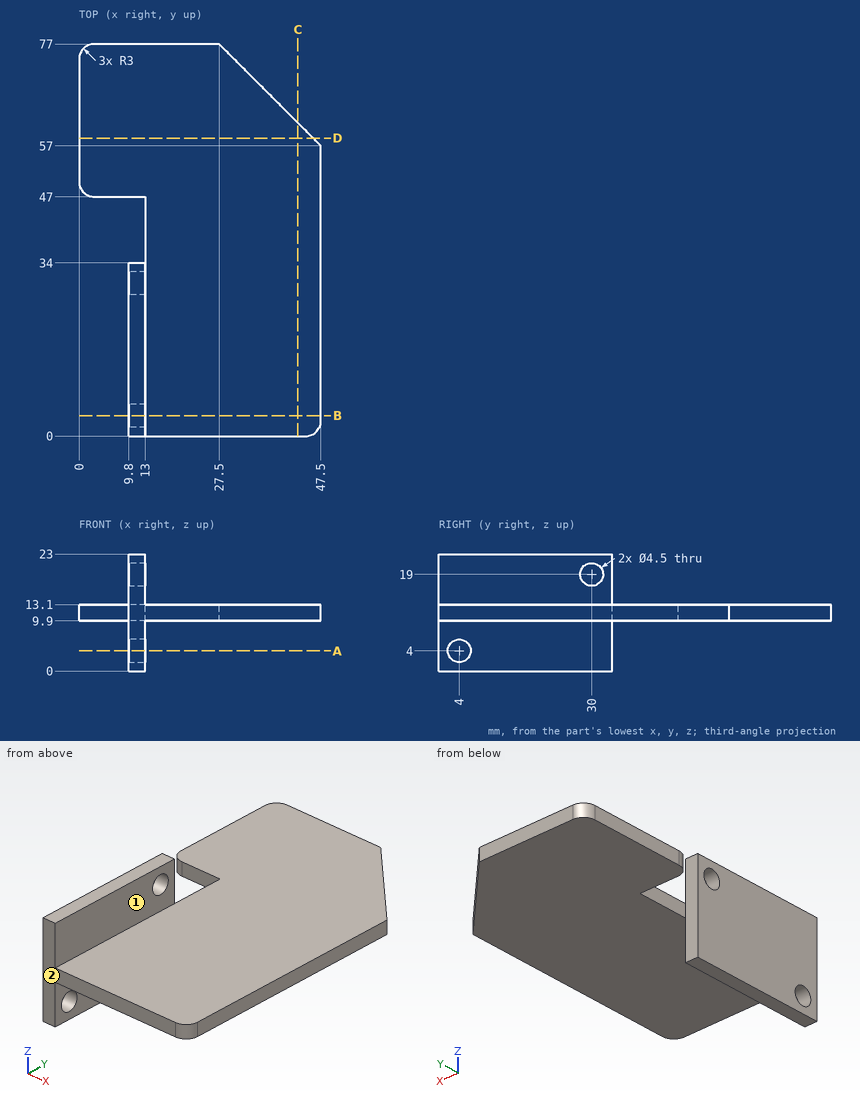
Print and shaded views of the part. All mm, measured from the part's lowest x, y and z. A direction names the side the tool comes from. Round coordinates to 2 decimals unless told otherwise and drop trailing zeros. Write each loop counter-clockwise with the first axis right and the second up, starting at its lowest first coordinate (ties: lowest second). Pieces come first, ordered by that corner, then holes. Notation, with made-up numbers: (7.25, 77) - (44.25, 77) arc R18 ccw to (44.25, 112) - close; hole circle Ø9 at (-37, 61). An arc over 180 degrees is marked (long way). One line per item, written item: value.
(1) 3-axis set-ups, long thin cutter, end or side, ignore diameter. For the marked faces 1 and 2: which of +Z, -Z, +X, -X, +Y, -Y reach the whole face in a straight line?
Values follow:
face 1: +Z, +X, +Y, -Y
face 2: +Z, -Z, +X, -X, -Y
(2) Drop flat-ended pins along their axis: P1, Ø3.5, axis at y = 30, z = 19, coming from the +X side; P2, Ø2.5, axis at y = 43.5, z = 11, coming from the -X side; P3, Ø5, axis at y = 16.5, z = 6.5, coming from the +X side; P4, Ø14.5, axis at x = 23, y = 35.5, coming from the -Z side. Give the stop position or say it passes through.
Values follow:
P1: passes through
P2: stops at x = 13
P3: stops at x = 13
P4: stops at z = 9.9
(3) Cut at A-A, the plane z = 4. Give the cut face in (x, y).
Values follow:
outline: (9.8, 0) - (13, 0) - (13, 1.75) - (9.8, 1.75) - close; (9.8, 6.25) - (13, 6.25) - (13, 34) - (9.8, 34) - close
(4) Wall check: probe 1 along Z at (x, y) = (11, 4); probe 2 along Y at (x, z) = (10.8, 19); probe 3 along Y at (x, z) = (10.75, 4). Give the ranges that are in metal, low to high.
Values follow:
probe 1: z = 0 to 1.75, 6.25 to 23
probe 2: y = 0 to 27.75, 32.25 to 34
probe 3: y = 0 to 1.75, 6.25 to 34
(5) Cut at D-D, the plane y = 58.5. Give the cut face in (x, z).
Values follow:
outline: (0, 9.9) - (46, 9.9) - (46, 13.1) - (0, 13.1) - close
(6) Cut at C-C, the plane x = 43. Give the cut face in (y, z), plus the area to 3 significant figures.
Values follow:
outline: (0, 9.9) - (61.5, 9.9) - (61.5, 13.1) - (0, 13.1) - close
area: 197 mm²
(7) Cut at B-B, the plane y = 4. Give the cut face in (x, z).
Values follow:
outline: (9.8, 0) - (13, 0) - (13, 1.75) - (9.8, 1.75) - close; (9.8, 6.25) - (13, 6.25) - (13, 9.9) - (47.5, 9.9) - (47.5, 13.1) - (13, 13.1) - (13, 23) - (9.8, 23) - close
